Geometry: final body of the model. Coordinates: model frame, mm. A direction names the side the tool comes from. Give positions to 0.01 mm unless a question says otherwise; leave off trailing zeros. Order: outer loops, then holes, each group sorted by start corner. A loop starts at its lowest first (then second) coordinate and runs counter-clockwise, first axis right, second up. Notation, with made-up numbers: (18.25, 42.5) -> (77.25, 42.5) arc R20 ccw to (77.25, 81.5) -> close; hole circle Ø1 at (-34, 49). An arc over 180 degrees is marked (long way). Answer in a Markdown table with one row per item. Add a question column.
Q1. Set-up query: faces 1 (the face through (1.16, -0.66, -0.96)), 2 (the face through (11.33, -11.3, 0.02)), 3 (the face through (0.728, 17.285, 0.018)), 4 (the face through (-14.43, 9.61, 0.02)), 5 (the face through (-13.599, -10.755, 0.018)). Return all of +Z, -Z, +X, -X, +Y, -Y with unobstructed straight access to the full face (end or side cutting, diameter ignored); none if empty.
Q2. Pull-direction query (X, two-part tool) for faces 6 (the face through (10.755, -13.599, 0.018)), 7 (the face through (4.649, -16.664, 0.018)), 8 (the face through (1.4, 0.7, -4.966)); classes: +X half, -X half, draft (parallel to the pull), parting line (faces both ways), or undercut.
Q3. Cut plane A-A on z = 2.5. Count the separate pieces of the cut face and the enclosed holes in it, and give its area (3 significant figures).
Q4. Contact query for flat-ended pins moving along their axis: P1, Ø1.5, axis at x = -1, z = 0, coming from the -Y side; P2, Ø6, axis at y = -14.5, z = 3.5, coming from the +X side; P3, Ø5.5, axis at x = 0, y = 6.95, coming from the -Z side; P4, Ø15, axis at x = 0, y = 0, coming from the -Z side. Output: stop coordinate, or through.
Q5. Line query: line 1 along Y through (x, z) = (0, 2.95) (1 decimal); line 2 along X through (y, z) = (2.5, -3.75); line 3 along Y through (x, z) = (0.5, -4.5). Output: solid intervals per line, ascending. Write a range as from..to.
Q6. Cut plane B-B on x = 7. Return the cut outline in (y, z), and give its area (3 significant figures).
from build123d import *

# Parameters (mm, degrees)
CUT_EXTRUDE2_DEPTH  = 17.78
SKETCH4_R           = 2.189434211
CUT_EXTRUDE3_DEPTH  = 1.6764
BOSS_EXTRUDE1_DEPTH = 2.54
SKETCH6_R           = 12.3698
CUT_EXTRUDE4_DEPTH  = 29.485557153


with BuildPart() as part:
    # Sketch1 → Revolve1 (revolve)
    with BuildSketch(Plane(origin=(0, 0, 0), x_dir=(0, 0, -1), z_dir=(1, 0, 0)), mode=Mode.PRIVATE) as revolve1_sk:
        Polygon((4.9657, 13.462), (1.27, 13.462), (1.27, 16.002), (-1.27, 16.002), (-1.27, 13.462), (-4.9657, 13.462), (-4.9657, 12.3698), (-0.8382, 12.3698), (-0.8382, 3.175), (-5.719832453, 3.175), (-5.719832453, 0), (0, 0), (14.625567547, 0), (14.625567547, 3.175), (0.8382, 3.175), (0.8382, 12.3698), (4.9657, 12.3698), align=None)
    revolve(revolve1_sk.sketch.rotate(Axis((0, 0, 0), (0, 0, -1)), 90), axis=Axis((0, 0, 0), (0, 0, -1)))

    # Sketch3 → Cut-Extrude2 (cut)
    with BuildSketch(Plane(origin=(0, 0, -14.625567547), x_dir=(-1, 0, 0), z_dir=(0, 0, -1))):
        Polygon((1.539793168, 0), (0.769896584, 1.3335), (-0.769896584, 1.3335), (-1.539793168, 0), (-0.769896584, -1.3335), (0.769896584, -1.3335), align=None)
    extrude(amount=-CUT_EXTRUDE2_DEPTH, mode=Mode.SUBTRACT)

    # Sketch4 → Cut-Extrude3 (cut)
    with BuildSketch(Plane(origin=(0, 0, -0.8382), x_dir=(-1, 0, 0), z_dir=(0, 0, -1))):
        with Locations((0, 6.954565789)):
            Circle(SKETCH4_R)
        with Locations((6.954565789, 0)):
            Circle(SKETCH4_R)
        with Locations((0, -6.954565789)):
            Circle(SKETCH4_R)
        with Locations((-6.954565789, 0)):
            Circle(SKETCH4_R)
    extrude(amount=-CUT_EXTRUDE3_DEPTH, mode=Mode.SUBTRACT)

    # Sketch5 → Boss-Extrude1 (add)
    with BuildSketch(Plane.XY.offset(1.27)):
        with BuildLine():
            ThreePointArc((-13.73725383, 8.206817971), (-12.945889944, 9.405739607), (-12.050192599, 10.528858548))
            Line((-12.050192599, 10.528858548), (-15.10552331, 10.974805092))
            Line((-15.10552331, 10.974805092), (-13.73725383, 8.206817971))
        make_face()
        with BuildLine():
            ThreePointArc((-10.528858548, 12.050192599), (-9.405739607, 12.945889944), (-8.206817971, 13.73725383))
            Line((-8.206817971, 13.73725383), (-10.974805092, 15.10552331))
            Line((-10.974805092, 15.10552331), (-10.528858548, 12.050192599))
        make_face()
        with BuildLine():
            ThreePointArc((-6.289825233, 14.714010417), (-4.944889944, 15.218806374), (-3.56010282, 15.600950994))
            Line((-3.56010282, 15.600950994), (-5.769796486, 17.757607659))
            Line((-5.769796486, 17.757607659), (-6.289825233, 14.714010417))
        make_face()
        with BuildLine():
            ThreePointArc((-1.4351, 15.937518376), (0, 16.002), (1.4351, 15.937518376))
            Line((1.4351, 15.937518376), (0, 18.671453646))
            Line((0, 18.671453646), (-1.4351, 15.937518376))
        make_face()
        with BuildLine():
            ThreePointArc((3.56010282, 15.600950994), (4.944889944, 15.218806374), (6.289825233, 14.714010417))
            Line((6.289825233, 14.714010417), (5.769796486, 17.757607659))
            Line((5.769796486, 17.757607659), (3.56010282, 15.600950994))
        make_face()
        with BuildLine():
            ThreePointArc((8.206817971, 13.73725383), (9.405739607, 12.945889944), (10.528858548, 12.050192599))
            Line((10.528858548, 12.050192599), (10.974805092, 15.10552331))
            Line((10.974805092, 15.10552331), (8.206817971, 13.73725383))
        make_face()
        with BuildLine():
            ThreePointArc((12.050192599, 10.528858548), (12.945889944, 9.405739607), (13.73725383, 8.206817971))
            Line((13.73725383, 8.206817971), (15.10552331, 10.974805092))
            Line((15.10552331, 10.974805092), (12.050192599, 10.528858548))
        make_face()
        with BuildLine():
            ThreePointArc((14.714010417, 6.289825233), (15.218806374, 4.944889944), (15.600950994, 3.56010282))
            Line((15.600950994, 3.56010282), (17.757607659, 5.769796486))
            Line((17.757607659, 5.769796486), (14.714010417, 6.289825233))
        make_face()
        with BuildLine():
            Line((18.671453646, 0), (16.002, 0))
            ThreePointArc((16.002, 0), (15.985871466, -0.718273954), (15.937518376, -1.4351))
            Line((15.937518376, -1.4351), (18.671453646, 0))
        make_face()
        with BuildLine():
            ThreePointArc((15.937518376, 1.4351), (15.985871466, 0.718273954), (16.002, 0))
            Line((16.002, 0), (18.671453646, 0))
            Line((18.671453646, 0), (15.937518376, 1.4351))
        make_face()
        with BuildLine():
            Line((17.757607659, -5.769796486), (15.600950994, -3.56010282))
            ThreePointArc((15.600950994, -3.56010282), (15.218806374, -4.944889944), (14.714010417, -6.289825233))
            Line((14.714010417, -6.289825233), (17.757607659, -5.769796486))
        make_face()
        with BuildLine():
            Line((15.10552331, -10.974805092), (13.73725383, -8.206817971))
            ThreePointArc((13.73725383, -8.206817971), (12.945889944, -9.405739607), (12.050192599, -10.528858548))
            Line((12.050192599, -10.528858548), (15.10552331, -10.974805092))
        make_face()
        with BuildLine():
            Line((10.974805092, -15.10552331), (10.528858548, -12.050192599))
            ThreePointArc((10.528858548, -12.050192599), (9.405739607, -12.945889944), (8.206817971, -13.73725383))
            Line((8.206817971, -13.73725383), (10.974805092, -15.10552331))
        make_face()
        with BuildLine():
            Line((5.769796486, -17.757607659), (6.289825233, -14.714010417))
            ThreePointArc((6.289825233, -14.714010417), (4.944889944, -15.218806374), (3.56010282, -15.600950994))
            Line((3.56010282, -15.600950994), (5.769796486, -17.757607659))
        make_face()
        with BuildLine():
            Line((0, -18.671453646), (1.4351, -15.937518376))
            ThreePointArc((1.4351, -15.937518376), (0, -16.002), (-1.4351, -15.937518376))
            Line((-1.4351, -15.937518376), (0, -18.671453646))
        make_face()
        with BuildLine():
            Line((-5.769796486, -17.757607659), (-3.56010282, -15.600950994))
            ThreePointArc((-3.56010282, -15.600950994), (-4.944889944, -15.218806374), (-6.289825233, -14.714010417))
            Line((-6.289825233, -14.714010417), (-5.769796486, -17.757607659))
        make_face()
        with BuildLine():
            Line((-10.974805092, -15.10552331), (-8.206817971, -13.73725383))
            ThreePointArc((-8.206817971, -13.73725383), (-9.405739607, -12.945889944), (-10.528858548, -12.050192599))
            Line((-10.528858548, -12.050192599), (-10.974805092, -15.10552331))
        make_face()
        with BuildLine():
            Line((-15.10552331, -10.974805092), (-12.050192599, -10.528858548))
            ThreePointArc((-12.050192599, -10.528858548), (-12.945889944, -9.405739607), (-13.73725383, -8.206817971))
            Line((-13.73725383, -8.206817971), (-15.10552331, -10.974805092))
        make_face()
        with BuildLine():
            Line((-17.757607659, -5.769796486), (-14.714010417, -6.289825233))
            ThreePointArc((-14.714010417, -6.289825233), (-15.218806374, -4.944889944), (-15.600950994, -3.56010282))
            Line((-15.600950994, -3.56010282), (-17.757607659, -5.769796486))
        make_face()
        with BuildLine():
            ThreePointArc((-15.937518376, -1.4351), (-16.002, 0), (-15.937518376, 1.4351))
            Line((-15.937518376, 1.4351), (-18.671453646, 0))
            Line((-18.671453646, 0), (-15.937518376, -1.4351))
        make_face()
        with BuildLine():
            ThreePointArc((-15.600950994, 3.56010282), (-15.218806374, 4.944889944), (-14.714010417, 6.289825233))
            Line((-14.714010417, 6.289825233), (-17.757607659, 5.769796486))
            Line((-17.757607659, 5.769796486), (-15.600950994, 3.56010282))
        make_face()
    extrude(amount=-BOSS_EXTRUDE1_DEPTH)

    # Sketch6 → Cut-Extrude4 (cut, through all)
    with BuildSketch(Plane(origin=(0, 0, -4.9657), x_dir=(-1, 0, 0), z_dir=(0, 0, -1))):
        with Locations(Location((0, 0, 0), (0, 0, 180))):
            Circle(SKETCH6_R)
    extrude(amount=CUT_EXTRUDE4_DEPTH, mode=Mode.SUBTRACT)


solid = part.part
Completed:
| question | item | result |
|---|---|---|
| 1 | face 1 | -Z |
| 1 | face 2 | +Z, -Z |
| 1 | face 3 | +Z, -Z, +Y |
| 1 | face 4 | +Z, -Z, -X |
| 1 | face 5 | +Z, -Z, -Y |
| 2 | face 6 | +X half |
| 2 | face 7 | undercut |
| 2 | face 8 | draft |
| 3 | separate pieces | 2 |
| 3 | enclosed holes | 2 |
| 3 | area | 114 mm² |
| 4 | P1 | stops at y = -18.2 |
| 4 | P2 | stops at x = 10.97 |
| 4 | P3 | stops at z = -0.84 |
| 4 | P4 | stops at z = -4.97 |
| 5 | line 1 | y = -13.5..-12.4, -3.2..-1.3, 1.3..3.2, 12.4..13.5 |
| 5 | line 2 | x = -13.23..-12.11, -1.96..1.96, 12.11..13.23 |
| 5 | line 3 | y = -13.45..-12.36, -3.14..-1.33, 1.33..3.14, 12.36..13.45 |
| 6 | outline | (-14.39, -1.27) -> (-11.5, -1.27) -> (-11.5, -4.97) -> (-10.2, -4.97) -> (-10.2, -0.84) -> (-2.19, -0.84) -> (-2.19, 0.84) -> (-10.2, 0.84) -> (-10.2, 4.97) -> (-11.5, 4.97) -> (-11.5, 1.27) -> (-14.39, 1.27) -> close; (2.19, -0.84) -> (10.2, -0.84) -> (10.2, -4.97) -> (11.5, -4.97) -> (11.5, -1.27) -> (14.39, -1.27) -> (14.39, 1.27) -> (11.5, 1.27) -> (11.5, 4.97) -> (10.2, 4.97) -> (10.2, 0.84) -> (2.19, 0.84) -> close |
| 6 | area | 67.4 mm² |
